Build history of the part. All positions in model axes, mm. A direction names the side the tool comes from. Give positions to 0.01 mm unless a question says otherwise; leave off trailing zeros. Write each loop counter-clockwise with the first axis right and the second up, starting at its lowest first coordinate (ties: lowest second). Pieces come first, ordered by that corner, then holes. Notation, with made-up numbers: M 15,36.25 L 22,36.25 A23 ccw 22,69.25 Z; hole C 49.5,-28.75 d3. An arc over 180 degrees is marked long. Return JSON: item names as keys, results as strings. Group by question number.
Q1. Wall check: probe 1 along X at (y, z) = (-3.75, -22); probe 2 along X at (y, z) = (-4.25, -19.5); probe 3 along Z at (x, y) = (-184, -4). Give the ranges that are in metal, low to high.
Q2. Band-saw the part on D-D, the plane x = -200. Give the cut face in (y, z).
Q3. Tool access for faces 1 (the flat face through (-191.36, -3.94, -36.63)), 2 (the flat face through (-193.702, -4, 11)), 3 (the flat face through (-141.966, -3.944, -33.375)), 4 (the flat face through (-176, 0, -23)), 5 (the flat face through (-163.702, -4, 11)): list every direction of +Z, -Z, +X, -X, +Y, -Y with a clear straight run to the whole face (end or side of a thin tool).
Q4. Band-saw the part on B-B, the plane y = -5. Give the cut face in (x, z) (3 decimals), then the cut area to 3 significant figures.
Q5. Pull direction X, two halves, no side cores. Call faces 6 (the flat face through (-166.389, -3.944, -36.433)), 7 (the cylindrical face through (-192.2, -3.94, 29.07)), 8 (the cylindrical face through (-165.128, -3.944, 28.993)): +X half, -X half, draft (parallel to the pull), parting line (faces both ways), or undercut.
Q6. Band-saw the part on A-A, the plane x = -183. Give the cut face in (y, z).
Q7. Flat gauge pin, fed straight in: pin 1 Ø17.5 at (x, z) = (-178.7, 18) entering from +Y. Where does the tip first touch, or does it go through?
Q8. Band-saw the part on C-C, the plane z = -19. Give the cut face in (x, y).
from build123d import *

# Parameters (mm, degrees)
F1_DEPTH = 8


with BuildPart() as f1:
    # F0 (on Front) → F1 (new body)
    with BuildSketch(Plane.XZ):
        with BuildLine():
            Line((-182.0272845483, 7.2368355937), (-178.701967001, 5.3169626126))
            Line((-178.701967001, 5.3169626126), (-175.3766494537, 7.2368355937))
            Line((-175.3766494537, 7.2368355937), (-172.0513319064, 1.4772166504))
            Line((-172.0513319064, 1.4772166504), (-163.701967001, -3.3432914252))
            Line((-163.701967001, -3.3432914252), (-163.701967001, 25.4964545369))
            ThreePointArc((-163.701967001, 25.4964545369), (-165.166433095, 29.0319884428), (-168.701967001, 30.4964545369))
            Line((-168.701967001, 30.4964545369), (-188.701967001, 30.4964545369))
            ThreePointArc((-188.701967001, 30.4964545369), (-192.2375009069, 29.0319884428), (-193.701967001, 25.4964545369))
            Line((-193.701967001, 25.4964545369), (-193.701967001, -3.3432914252))
            Line((-193.701967001, -3.3432914252), (-185.3526020956, 1.4772166504))
            Line((-185.3526020956, 1.4772166504), (-182.0272845483, 7.2368355937))
        make_face()
        with BuildLine():
            ThreePointArc((-167.776967001, 17.9964545369), (-170.9768254165, 10.2713129525), (-178.701967001, 7.0714545369))
            ThreePointArc((-178.701967001, 7.0714545369), (-186.4271085854, 25.7215961214), (-167.776967001, 17.9964545369))
        make_face(mode=Mode.SUBTRACT)
        with BuildLine():
            Line((-160.3766494537, -18.7439265199), (-163.701967001, -20.6637995009))
            Line((-163.701967001, -20.6637995009), (-163.701967001, -24.5035454631))
            Line((-163.701967001, -24.5035454631), (-170.3526020956, -24.5035454631))
            Line((-170.3526020956, -24.5035454631), (-178.701967001, -29.3240535388))
            Line((-178.701967001, -29.3240535388), (-153.726014359, -43.7439265199))
            ThreePointArc((-153.726014359, -43.7439265199), (-149.9319191335, -44.2434286324), (-146.8958873401, -41.9137995009))
            Line((-146.8958873401, -41.9137995009), (-136.8958873401, -24.5932914252))
            ThreePointArc((-136.8958873401, -24.5932914252), (-136.3963852276, -20.7991961997), (-138.726014359, -17.7631644063))
            Line((-138.726014359, -17.7631644063), (-163.701967001, -3.3432914252))
            Line((-163.701967001, -3.3432914252), (-163.701967001, -12.9843075766))
            Line((-163.701967001, -12.9843075766), (-160.3766494537, -18.7439265199))
        make_face()
        with BuildLine():
            ThreePointArc((-141.7962048874, -27.0035454631), (-155.5488029552, -37.5562851153), (-162.1825324238, -21.5410454631))
            ThreePointArc((-162.1825324238, -21.5410454631), (-149.8936068197, -16.4508058109), (-141.7962048874, -27.0035454631))
        make_face(mode=Mode.SUBTRACT)
        with BuildLine():
            Line((-193.701967001, -24.5035454631), (-193.701967001, -20.6637995009))
            Line((-193.701967001, -20.6637995009), (-197.0272845483, -18.7439265199))
            Line((-197.0272845483, -18.7439265199), (-193.701967001, -12.9843075766))
            Line((-193.701967001, -12.9843075766), (-193.701967001, -3.3432914252))
            Line((-193.701967001, -3.3432914252), (-218.6779196429, -17.7631644063))
            ThreePointArc((-218.6779196429, -17.7631644063), (-221.0075487743, -20.7991961997), (-220.5080466618, -24.5932914252))
            Line((-220.5080466618, -24.5932914252), (-210.5080466618, -41.9137995009))
            ThreePointArc((-210.5080466618, -41.9137995009), (-207.4720148684, -44.2434286324), (-203.6779196429, -43.7439265199))
            Line((-203.6779196429, -43.7439265199), (-178.701967001, -29.3240535388))
            Line((-178.701967001, -29.3240535388), (-187.0513319064, -24.5035454631))
            Line((-187.0513319064, -24.5035454631), (-193.701967001, -24.5035454631))
        make_face()
        with BuildLine():
            ThreePointArc((-193.7577291145, -27.0035454631), (-215.2354687667, -29.8311435308), (-195.2214015781, -21.5410454631))
            ThreePointArc((-195.2214015781, -21.5410454631), (-194.1299894623, -24.1759473953), (-193.7577291145, -27.0035454631))
        make_face(mode=Mode.SUBTRACT)
        Polygon((-193.701967001, -12.9843075766), (-185.3526020956, 1.4772166504), (-193.701967001, -3.3432914252), align=None)
        Polygon((-163.701967001, -3.3432914252), (-172.0513319064, 1.4772166504), (-163.701967001, -12.9843075766), align=None)
        Polygon((-178.701967001, -29.3240535388), (-170.3526020956, -24.5035454631), (-187.0513319064, -24.5035454631), align=None)
        with BuildLine():
            ThreePointArc((-188.1632945373, -17.4660454631), (-188.1632945373, -6.5410454631), (-178.701967001, -1.0785454631))
            Line((-178.701967001, -1.0785454631), (-178.701967001, 5.3169626126))
            Line((-178.701967001, 5.3169626126), (-185.3526020956, 1.4772166504))
            Line((-185.3526020956, 1.4772166504), (-193.701967001, -12.9843075766))
            Line((-193.701967001, -12.9843075766), (-193.701967001, -20.6637995009))
            Line((-193.701967001, -20.6637995009), (-188.1632945373, -17.4660454631))
        make_face()
        with BuildLine():
            ThreePointArc((-178.701967001, -1.0785454631), (-170.9768254165, -4.2784038786), (-167.776967001, -12.0035454631))
            ThreePointArc((-167.776967001, -12.0035454631), (-168.1492273488, -14.8311435308), (-169.2406394646, -17.4660454631))
            Line((-169.2406394646, -17.4660454631), (-163.701967001, -20.6637995009))
            Line((-163.701967001, -20.6637995009), (-163.701967001, -12.9843075766))
            Line((-163.701967001, -12.9843075766), (-172.0513319064, 1.4772166504))
            Line((-172.0513319064, 1.4772166504), (-178.701967001, 5.3169626126))
            Line((-178.701967001, 5.3169626126), (-178.701967001, -1.0785454631))
        make_face()
        Polygon((-175.3766494537, 7.2368355937), (-178.701967001, 5.3169626126), (-172.0513319064, 1.4772166504), align=None)
        Polygon((-185.3526020956, 1.4772166504), (-178.701967001, 5.3169626126), (-182.0272845483, 7.2368355937), align=None)
        with BuildLine():
            Line((-163.701967001, -20.6637995009), (-169.2406394646, -17.4660454631))
            ThreePointArc((-169.2406394646, -17.4660454631), (-178.701967001, -22.9285454631), (-188.1632945373, -17.4660454631))
            Line((-188.1632945373, -17.4660454631), (-193.701967001, -20.6637995009))
            Line((-193.701967001, -20.6637995009), (-187.0513319064, -24.5035454631))
            Line((-187.0513319064, -24.5035454631), (-170.3526020956, -24.5035454631))
            Line((-170.3526020956, -24.5035454631), (-163.701967001, -20.6637995009))
        make_face()
        Polygon((-163.701967001, -12.9843075766), (-163.701967001, -20.6637995009), (-160.3766494537, -18.7439265199), align=None)
        Polygon((-163.701967001, -24.5035454631), (-163.701967001, -20.6637995009), (-170.3526020956, -24.5035454631), align=None)
        Polygon((-187.0513319064, -24.5035454631), (-193.701967001, -20.6637995009), (-193.701967001, -24.5035454631), align=None)
        Polygon((-197.0272845483, -18.7439265199), (-193.701967001, -20.6637995009), (-193.701967001, -12.9843075766), align=None)
    extrude(amount=F1_DEPTH)


solid = f1.part
From the geometry:
{
 "1": {"probe 1": "x = -221.18 to -214.39, -194.97 to -183.11, -174.29 to -162.43, -143.01 to -136.23", "probe 2": "x = -220.45 to -212.62, -196.74 to -186.65, -170.75 to -160.66, -144.78 to -136.95", "probe 3": "z = -32.38 to -21.56, -2.45 to 8.44, 27.55 to 30.5"},
 "2": {"outline": "M -8,-41.62 L 0,-41.62 L 0,-36.87 L -8,-36.87 Z; M -8,-17.13 L 0,-17.13 L 0,-6.98 L -8,-6.98 Z"},
 "3": {"face 1": "-Z, +Y, -Y", "face 2": "+Z, -X, +Y, -Y", "face 3": "-Z, +X, +Y, -Y", "face 4": "+Z, -Z, +X, -X, +Y", "face 5": "+Z, +X, +Y, -Y"},
 "4": {"outline": "M -220.508,-24.593 L -210.508,-41.914 A5 ccw -203.678,-43.744 L -178.702,-29.324 L -153.726,-43.744 A5 ccw -146.896,-41.914 L -136.896,-24.593 A5 ccw -138.726,-17.763 L -163.702,-3.343 L -163.702,25.496 A5 ccw -168.702,30.496 L -188.702,30.496 A5 ccw -193.702,25.496 L -193.702,-3.343 L -218.678,-17.763 A5 ccw Z; hole C -204.683,-27.004 d21.85; hole C -178.702,-12.004 d21.85; hole C -178.702,17.996 d21.85; hole C -152.721,-27.004 d21.85", "area": "1,900 mm^2"},
 "5": {"face 6": "undercut", "face 7": "-X half", "face 8": "+X half"},
 "6": {"outline": "M -8,-31.81 L 0,-31.81 L 0,-22.05 L -8,-22.05 Z; M -8,-1.96 L 0,-1.96 L 0,7.95 L -8,7.95 Z; M -8,28.04 L 0,28.04 L 0,30.5 L -8,30.5 Z"},
 "7": {"pin 1": "passes through"},
 "8": {"outline": "M -220.11,-8 L -212.12,-8 L -212.12,0 L -220.11,0 Z; M -197.25,-8 L -187.09,-8 L -187.09,0 L -197.25,0 Z; M -170.31,-8 L -160.16,-8 L -160.16,0 L -170.31,0 Z; M -145.28,-8 L -137.3,-8 L -137.3,0 L -145.28,0 Z"}
}
